Here's how the part is built. I have some questions about the finished solid (model axes, mm). A direction names the side the tool comes from. Round coordinates to 2 decimals unless told otherwise and drop trailing zeros. Loops run counter-clockwise (first coordinate to the right, second up) from the corner with the lowest first, then second, coordinate; pieces in that order, holes last. Notation, with made-up numbers: (70.25, 85) -> (82.25, 85) arc R25 cw to (82.25, 99) -> close; hole circle Ø6 at (35.5, -28.75). An arc over 180 degrees is marked (long way). Use one line per item in the form item = value. Start each with the question number.
Item 1: If I drill on L1, parallel to Z at x = 140.97, y = 3.5; L2, parallel to X at y = 5, z = -59; L3, parallel to X at y = 31.5, z = -67.5, over which ranges is the centre line in solid material (lowest first)? Write a range as [from, to].
Item 2: For faces 5 (the face through (81, 40, -52)), 6 (the face through (159, 20, -100.33)), 7 (the face through (2.921, 21, -51)), 8 (the face through (0, 1, -55)), 9 (the face through (159, 23.622, -46)), which set-ups out of +Z, -Z, +X, -X, +Y, -Y let a thin tool reach every point of the face, with its end or its side?
Item 3: Thinking about a two-plate mould opening in Z: for faces 1 (the face through (63, 20, 0)), 2 (the face through (81, 0, -52)), 3 (the face through (159, 1.27, -90)), 4 (the face through (159, 12, -80.264)), which applies, released by +Z, released by -Z, zero draft, split by the parting line, or undercut?
Item 4: If we section it at B-B (y = 26.5): Write out the boundary of the cut face in (x, z), then the cut area to 3 significant figures.
Item 5: If we section it at C-C (y = 5.5): Write out the boundary of the cut face in (x, z).
Item 6: I'm going to push flat-ended pins straight in: pin 1 Ø6 at (x, z) = (161.5, -37.5) entering from +Y; pin 2 Ø2.5 at (x, y) = (1.5, 12.5) entering from +Z; pin 3 Ø1.3 at (x, z) = (160, -21) entering from +Y. Where does each tip first touch, or does it pass through?
Item 7: If we section it at A-A (z = -77): Write out the boundary of the cut face in (x, y).
```python
from build123d import *

# Parameters (mm, degrees)
SKETCH1_W           = 165.1
SKETCH1_H           = 101.6
BOSS_EXTRUDE1_DEPTH = 40
SKETCH2_W           = 100.33
SKETCH2_H           = 38.73
CUT_EXTRUDE1_DEPTH  = 11.43
SKETCH3_W           = 100.33
SKETCH3_H           = 38.73
CUT_EXTRUDE2_DEPTH  = 2.921
SKETCH4_W           = 11.43
SKETCH4_H           = 68.58
BOSS_EXTRUDE2_DEPTH = 22.352
CUT_EXTRUDE3_DEPTH  = 22.352
SKETCH6_R           = 1.27
CUT_EXTRUDE4_DEPTH  = 10.16
SKETCH7_W           = 11.43
SKETCH7_H           = 2.54
CUT_EXTRUDE5_DEPTH  = 12.7


with BuildPart() as part:
    # Sketch1 → Boss-Extrude1 (new body)
    with BuildSketch(Plane(origin=(0, 0, 0), x_dir=(1, 0, 0), z_dir=(0, 1, 0))):
        with Locations((82.55, 50.8)):
            Rectangle(SKETCH1_W, SKETCH1_H)
    extrude(amount=BOSS_EXTRUDE1_DEPTH)

    # Sketch2 → Cut-Extrude1 (cut)
    with BuildSketch(Plane(origin=(165.1, 0, 0), x_dir=(0, 0, -1), z_dir=(1, 0, 0))):
        with Locations((50.165, 20.635)):
            Rectangle(SKETCH2_W, SKETCH2_H)
    extrude(amount=-CUT_EXTRUDE1_DEPTH, mode=Mode.SUBTRACT)

    # Sketch3 → Cut-Extrude2 (cut)
    with BuildSketch(Plane.ZY):
        with Locations((-50.165, 20.635)):
            Rectangle(SKETCH3_W, SKETCH3_H)
    extrude(amount=-CUT_EXTRUDE2_DEPTH, mode=Mode.SUBTRACT)

    # Sketch4 → Boss-Extrude2 (add)
    with BuildSketch(Plane(origin=(0, 1.27, 0), x_dir=(1, 0, 0), z_dir=(0, 1, 0))):
        with Locations((159.385, 45.974)):
            Rectangle(SKETCH4_W, SKETCH4_H)
    extrude(amount=BOSS_EXTRUDE2_DEPTH)

    # Sketch5 → Cut-Extrude3 (cut)
    with BuildSketch(Plane(origin=(0, 1.27, 0), x_dir=(1, 0, 0), z_dir=(0, 1, 0))):
        with BuildLine():
            Line((0, 8.255), (0, 5.08))
            Line((0, 5.08), (4.0005, 5.08))
            ThreePointArc((4.0005, 5.08), (5.588, 6.6675), (4.0005, 8.255))
            Line((4.0005, 8.255), (0, 8.255))
        make_face()
        with BuildLine():
            Line((165.1, 92.837), (165.1, 96.012))
            Line((165.1, 96.012), (161.0995, 96.012))
            ThreePointArc((161.0995, 96.012), (159.512, 94.4245), (161.0995, 92.837))
            Line((161.0995, 92.837), (165.1, 92.837))
        make_face()
    extrude(amount=-CUT_EXTRUDE3_DEPTH, mode=Mode.SUBTRACT)

    # Sketch6 → Cut-Extrude4 (cut)
    with BuildSketch(Plane.XZ):
        with Locations((63.246, -65.278)):
            Circle(SKETCH6_R)
        with Locations((140.97, -65.278)):
            Circle(SKETCH6_R)
    extrude(amount=-CUT_EXTRUDE4_DEPTH, mode=Mode.SUBTRACT)

    # Sketch7 → Cut-Extrude5 (cut)
    with BuildSketch(Plane(origin=(0, 23.622, 0), x_dir=(1, 0, 0), z_dir=(0, 1, 0))):
        with Locations((159.385, 71.374)):
            Rectangle(SKETCH7_W, SKETCH7_H)
        with Locations((159.385, 61.214)):
            Rectangle(SKETCH7_W, SKETCH7_H)
        with Locations((159.385, 51.054)):
            Rectangle(SKETCH7_W, SKETCH7_H)
        with Locations((159.385, 40.894)):
            Rectangle(SKETCH7_W, SKETCH7_H)
        with Locations((159.385, 30.734)):
            Rectangle(SKETCH7_W, SKETCH7_H)
        with Locations((159.385, 20.574)):
            Rectangle(SKETCH7_W, SKETCH7_H)
    extrude(amount=-CUT_EXTRUDE5_DEPTH, mode=Mode.SUBTRACT)


solid = part.part
```
Values found:
q1.L1 = [-101.6, -66.55], [-64.01, 0]
q1.L2 = [2.92, 165.1]
q1.L3 = [2.92, 153.67]
q2.face_5 = +Z, -Z, +X, -X, +Y
q2.face_6 = +X, +Y
q2.face_7 = +Z, -X, +Y
q2.face_8 = +Z, -Z, -X, +Y, -Y
q2.face_9 = +Z, +X, +Y
q3.face_1 = released by +Z
q3.face_2 = zero draft
q3.face_3 = undercut
q3.face_4 = undercut
q4.outline = (0, -101.6) -> (165.1, -101.6) -> (165.1, -100.33) -> (153.67, -100.33) -> (153.67, 0) -> (2.92, 0) -> (2.92, -100.33) -> (0, -100.33) -> close
q4.area = 15,300 mm2
q5.outline = (0, -101.6) -> (165.1, -101.6) -> (165.1, -100.33) -> (153.67, -100.33) -> (153.67, -80.26) -> (165.1, -80.26) -> (165.1, -11.68) -> (153.67, -11.68) -> (153.67, 0) -> (2.92, 0) -> (2.92, -100.33) -> (0, -100.33) -> close; hole circle Ø2.54 at (63.25, -65.28); hole circle Ø2.54 at (140.97, -65.28)
q6.pin_1 = 23.62
q6.pin_2 = -100.33
q6.pin_3 = 10.92
q7.outline = (0, 0) -> (165.1, 0) -> (165.1, 23.62) -> (153.67, 23.62) -> (153.67, 40) -> (2.92, 40) -> (2.92, 1.27) -> (0, 1.27) -> close
